from build123d import *

# Parameters (mm, degrees)
SKETCH1_W           = 40.132
SKETCH1_H           = 18.1737
PCB_BOARD_DEPTH     = 1.524
SKETCH2_W           = 6.096
SKETCH2_H           = 6.096
BOSS_EXTRUDE1_DEPTH = 1.27
SKETCH3_R           = 3.91795
BOSS_EXTRUDE2_DEPTH = 120
SKETCH4_R           = 1.476375
CUT_EXTRUDE1_DEPTH  = 1.524


with BuildPart() as part:
    # Sketch1 → PCB board (new body)
    with BuildSketch(Plane(origin=(0, 0, 0), x_dir=(1, 0, 0), z_dir=(0, 1, 0))):
        Rectangle(SKETCH1_W, SKETCH1_H)
    extrude(amount=PCB_BOARD_DEPTH)

    # Sketch2 → Boss-Extrude1 (add)
    with BuildSketch(Plane.ZY.offset(20.066)):
        with Locations((6.03885, 3.048)):
            Rectangle(SKETCH2_W, SKETCH2_H)
    extrude(amount=BOSS_EXTRUDE1_DEPTH)

    # Sketch3 → Boss-Extrude2 (add)
    with BuildSketch(Plane.ZY.offset(21.336)):
        with Locations((6.03885, 3.048)):
            Circle(SKETCH3_R)
    extrude(amount=BOSS_EXTRUDE2_DEPTH)

    # Sketch4 → Cut-Extrude1 (cut)
    with BuildSketch(Plane(origin=(0, 1.524, 0), x_dir=(1, 0, 0), z_dir=(0, 1, 0))):
        with Locations((-17.776825, 0)):
            Circle(SKETCH4_R)
        with Locations((18.437225, 0)):
            Circle(SKETCH4_R)
    extrude(amount=-CUT_EXTRUDE1_DEPTH, mode=Mode.SUBTRACT)


solid = part.part
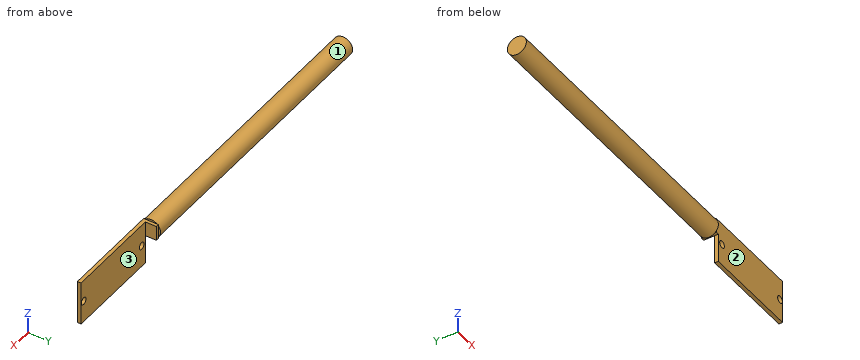
Geometry check sheet. Reference: the model listing, model coordinates, mm. Face numbers are marked on the shaded views. A direction names the side the tool comes from. Coordinates: 2 decimals unless noted, no trailing zeros. Loops run counter-clockwise (first coordinate to the right, second up) from the corner with the lowest first, then second, coordinate; pieces in that order, holes last. Notation, with made-up numbers: (31, 16.25) - (63, 16.25) arc R23 ccw to (63, 53.25) - close; hole circle Ø5 at (47, 21.25). An arc over 180 degrees is marked (long way). Use one line per item in the form item = value. Start each with the question number.
Item 1: Thickness scan on probe 1 along X at (y, z) = (0.55, 0); probe 2 along Z at (x, y) = (-18, 1); probe 3 along X at (y, z) = (4, 4.25). Record the ranges inside material, lowest first.
Item 2: Gauge pin test, flat ends, axial feed: pin 1 (0.6 mm diameter, centred on x = -21, y = 4.5, fed in from -Z); pin 2 (3.5 mm diameter, centred on y = 5, z = 6, fed in from +X); pin 3 (0.7 mm diameter, centred on y = -0.5, z = 5, fed in from +X). Record the tip position at first contact, or that the pin passes through.
Item 3: Section check A-A, the plane z = 0. Enter the section's corners in (x, y), and give its area (3 significant figures).
Item 4: Tool access check on the marked faces 1, 2 and 3. Record the directions out of +Z, -Z, +X, -X, +Y, -Y that give a thin tool (end or side, any length) a straight path to the whole face; none if there is none.
Item 5: Section check B-B, the plane x = -131. Enter the section's corners in (y, z), and give its area (3 significant figures).
Computed:
q1.probe_1 = -20.07 to -19.25, -16.3 to 16.96, 19.91 to 20.07
q1.probe_2 = -9.09 to -1.46, 1.46 to 9.09
q1.probe_3 = -141.34 to -20.07
q2.pin_1 = 2.99
q2.pin_2 = -20.07
q2.pin_3 = -21.34
q3.outline = (-20.07, 0) - (-19.25, 0) - (-19.25, 1.52) - (-20.07, 1.52) - close; (-16.3, 0) - (16.96, 0) - (16.96, 1.52) - (-16.3, 1.52) - close; (19.91, 0) - (20.07, 0) - (20.07, 1.52) - (19.91, 1.52) - close
q3.area = 52.2 mm2
q4.face_1 = -X
q4.face_2 = +Z, -Z, +X, -Y
q4.face_3 = +Z, -Z, +X, +Y
q5.outline = circle Ø7.84 at (3.05, 6.04)
q5.area = 48.2 mm2
